For this review, take the finished solid that the model builds, in its own axes (mm). A direction names the side the tool comes from. Give positions to 0.01 mm unless a question says otherwise; leave off trailing zeros. Write each loop counter-clockwise with the first axis right and the second up, starting at its lowest first coordinate (ties: lowest second). Pieces come first, ordered by that corner, then holes. Notation, with made-up numbers: M 5.25,15 L 63.25,15 A16 cw 63.25,30 Z; hole C 72,89 d1. An arc over 180 degrees is marked long. Use one line per item in the form item = value. Start each with the question number.
Q1. Consider section D-D on y = 34. Write out the cut boundary in (x, z), and give its area (3 significant figures).
Q2. For probe 1 along Y at (x, z) = (-6, -10.75); probe 2 along Y at (x, z) = (-4.5, -10.5); probe 3 along X at (y, z) = (54.5, -0.25), list the stretches that pass through material, from the lowest coordinate up. Write a range as [from, to].
Q3. Consider section C-C on y = 50. Write out the cut boundary in (x, z).
Q4. Tool access review of faces 1 (the flat face through (9, -3, -1)), 2 (the cylindrical face through (-3.417, 50.479, -0.759)), 3 (the flat face through (-9, -3, 1)), 4 (the flat face through (-11.8, -3, 0)), 5 (the flat face through (-6.8, -3, 0)): name each direction out of +Z, -Z, +X, -X, +Y, -Y from which nothing blocks a thin tool from reaching the whole face with its end or side.
Q5. Consider section B-B on z = 0. Write out the cut boundary in (x, y), and give its area (3 significant figures).
Q6. Consider section A-A on x = 0. Write out the cut boundary in (y, z).
Q7. Mouldability with a two-part tool opening along X and no side actions: class faces 6 (the flat face through (9, -3, 1)), 7 (the flat face through (11.8, -3, 0)), 8 (the flat face through (6.8, -3, 0)) as released by +X, released by -X, zero draft, split by the parting line, or undercut.
Q8. Clearance check with flat-ended pins moving along their axes: pin 1 Ø4 at (x, y) = (10, -2.5) entering from -Z; pin 2 Ø1 at (x, z) = (-9, -4.5) entering from +Y; pin 3 Ø1.5 at (x, y) = (-8, -3.5) entering from +Z. State where each tip first meets the part, or that it passes through.
```python
from build123d import *

# Parameters (mm, degrees)
ESBO_O1_R                = 12.5
RESSALTO_EXTRUS_O1_DEPTH = 31
FILETE1_R                = 1
ESBO_O2_R                = 12.5
RESSALTO_EXTRUS_O2_DEPTH = 18
ESBO_O3_W                = 5
ESBO_O3_H                = 2
RESSALTO_EXTRUS_O3_DEPTH = 6
ESBO_O5_R                = 3.5
RESSALTO_EXTRUS_O4_DEPTH = 3
RESSALTO_EXTRUS_O5_DEPTH = 10


with BuildPart() as part:
    # Esboço1 → Ressalto-extrusão1 (new body)
    with BuildSketch(Plane(origin=(0, 0, 0), x_dir=(1, 0, 0), z_dir=(0, 1, 0))):
        with Locations(Location((0, 0, 0), (0, 0, 270))):
            Circle(ESBO_O1_R)
    extrude(amount=RESSALTO_EXTRUS_O1_DEPTH)

    # Filete1
    filete1_edges = [part.edges().sort_by_distance(p)[0] for p in [
        (0, 31, -12.5),
    ]]
    fillet(filete1_edges, radius=FILETE1_R)

    # Esboço2 → Ressalto-extrusão2 (add)
    with BuildSketch(Plane(origin=(0, 31, 0), x_dir=(1, 0, 0), z_dir=(0, 1, 0))):
        with Locations(Location((0, 0, 0), (0, 0, 270))):
            Circle(ESBO_O2_R)
    extrude(amount=RESSALTO_EXTRUS_O2_DEPTH)

    # Esboço3 → Ressalto-extrusão3 (add)
    with BuildSketch(Plane.XZ):
        with Locations((9.3, 0)):
            Rectangle(ESBO_O3_W, ESBO_O3_H)
        with Locations((-9.3, 0)):
            Rectangle(ESBO_O3_W, ESBO_O3_H)
    extrude(amount=RESSALTO_EXTRUS_O3_DEPTH)

    # Esboço5 → Ressalto-extrusão4 (add)
    with BuildSketch(Plane(origin=(0, 49, 0), x_dir=(1, 0, 0), z_dir=(0, 1, 0))):
        with Locations(Location((0, 0, 0), (0, 0, 270))):
            Circle(ESBO_O5_R)
    extrude(amount=RESSALTO_EXTRUS_O4_DEPTH)

    # Esboço6 → Ressalto-extrusão5 (add)
    with BuildSketch(Plane(origin=(0, 52, 0), x_dir=(1, 0, 0), z_dir=(0, 1, 0))):
        with BuildLine():
            ThreePointArc((-1.732050808, 1), (0, -2), (1.732050808, 1))
            Line((1.732050808, 1), (-1.732050808, 1))
        make_face()
    extrude(amount=RESSALTO_EXTRUS_O5_DEPTH)


solid = part.part
```
Working result:
q1.outline = C 0,0 d25
q1.area = 491 mm²
q2.probe_1 = [0, 30.58], [31, 49]
q2.probe_2 = [0, 49]
q2.probe_3 = [-1.98, 1.98]
q3.outline = C 0,0 d7
q4.face_1 = -Z, +X, -X, -Y
q4.face_2 = +Y
q4.face_3 = +Z, +X, -X, -Y
q4.face_4 = +Z, -Z, -X, -Y
q4.face_5 = +Z, -Z, -Y
q5.outline = M -12.5,0 L -11.8,0 L -11.8,-6 L -6.8,-6 L -6.8,0 L 6.8,0 L 6.8,-6 L 11.8,-6 L 11.8,0 L 12.5,0 L 12.5,30 A1 ccw 11.5,31 L 12.5,31 L 12.5,49 L 3.5,49 L 3.5,52 L 2,52 L 2,62 L -2,62 L -2,52 L -3.5,52 L -3.5,49 L -12.5,49 L -12.5,31 L -11.5,31 A1 ccw -12.5,30 Z
q5.area = 1,350 mm²
q6.outline = M 0,-12.5 L 30,-12.5 A1 ccw 31,-11.5 L 31,-12.5 L 49,-12.5 L 49,-3.5 L 52,-3.5 L 52,-1 L 62,-1 L 62,2 L 52,2 L 52,3.5 L 49,3.5 L 49,12.5 L 31,12.5 L 31,11.5 A1 ccw 30,12.5 L 0,12.5 Z
q7.face_6 = zero draft
q7.face_7 = released by +X
q7.face_8 = undercut
q8.pin_1 = -1
q8.pin_2 = 49
q8.pin_3 = 1
